Model file for the job. Use its own axes, mm. Give positions to 0.01 mm unless a question says otherwise; leave off trailing zeros. Loops run counter-clockwise (first coordinate to the right, second up) from the corner with the lowest first, then second, coordinate; pieces in that order, holes last. Notation, with made-up numbers: (-23, 56) - (3, 56) arc R26 ccw to (3, 91) - close; hole circle Ø10 at (20.5, -32). An arc over 180 degrees is marked (long way). Answer as CSV lines item,"result". Start each with the question number.
Item 1: Pull direction Y, two halves, no side cores. Call faces 1 (the cylindrical face through (0, -1, 1)), 2 (the flat face through (0, -2, 121)), 3 (the cylindrical face through (0.867, -3.905, 61.34)), 4 (the cylindrical face through (0, -1, 120)): pulls with the +Y half, pulls with the -Y half, needs draft (parallel to the pull), parting line crosses it, or undercut.
Item 2: Pin check, flat tips, straight feed: pin 1 (2 mm diameter, centred on y = 3, z = 22.5, fed in from +X); pin 2 (1 mm diameter, centred on x = -2.5, z = 88.5, fed in from -Y); pin 3 (1 mm diameter, centred on y = -3, z = 99, fed in from -X). Stop position of each tip, or through.
Item 3: Saw through at A-A on z = 64.5. Give the cut face in (x, y), plus the area to 3 significant figures.
Item 4: Drill centre lines: L1, parallel to Y at x = 0, z = 1.15; L2, parallel to Y at x = -0.25, z = 104.5. Where is each one in solid material? Low to high. Write a range as from..to.
from build123d import *

# Parameters (mm, degrees)
CHAMFER1_SIZE         = 0.5
CHAMFER2_SIZE         = 0.3
CHAMFER2_SIZE2        = 0.173205081
CHAMFER2_PART_2_SIZE  = 0.3
CHAMFER2_PART_2_SIZE2 = 0.173205081
CHAMFER2_PART_3_SIZE  = 0.3
CHAMFER2_PART_3_SIZE2 = 0.173205081
CHAMFER2_PART_4_SIZE  = 0.3
CHAMFER2_PART_4_SIZE2 = 0.173205081


with BuildPart() as part:
    # Sketch1 → Revolve1 (revolve)
    with BuildSketch(Plane(origin=(0, 0, 0), x_dir=(1, 0, 0), z_dir=(0, 1, 0))):
        Polygon((-1, 0), (-4, 0), (-4, -121), (-1, -121), (-1, -119), (0, -119), (0, -2), (-1, -2), align=None)
    revolve(axis=Axis((0, 0, 119), (0, 0, -1)))

    # Chamfer1
    chamfer1_edges = [part.edges().sort_by_distance(p)[0] for p in [
        (4, 0, 121),
        (4, 0, 0),
    ]]
    chamfer(chamfer1_edges, length=CHAMFER1_SIZE)

    # Chamfer2
    chamfer2_edges = [part.edges().sort_by_distance(p)[0] for p in [
        (1, 0, 2),
    ]]
    chamfer2_side = [part.faces().sort_by_distance(p)[0] for p in [
        (0, 0, 2),
    ]]
    chamfer(chamfer2_edges, length=CHAMFER2_SIZE, length2=CHAMFER2_SIZE2, reference=chamfer2_side[0])

    # Chamfer2 part 2
    chamfer2_part_2_edges = [part.edges().sort_by_distance(p)[0] for p in [
        (1, 0, 119),
    ]]
    chamfer2_part_2_side = [part.faces().sort_by_distance(p)[0] for p in [
        (1, 0, 120),
    ]]
    chamfer(chamfer2_part_2_edges, length=CHAMFER2_PART_2_SIZE, length2=CHAMFER2_PART_2_SIZE2, reference=chamfer2_part_2_side[0])

    # Chamfer2 part 3
    chamfer2_part_3_edges = [part.edges().sort_by_distance(p)[0] for p in [
        (1, 0, 121),
    ]]
    chamfer2_part_3_side = [part.faces().sort_by_distance(p)[0] for p in [
        (3.401005051, 0, 121),
    ]]
    chamfer(chamfer2_part_3_edges, length=CHAMFER2_PART_3_SIZE, length2=CHAMFER2_PART_3_SIZE2, reference=chamfer2_part_3_side[0])

    # Chamfer2 part 4
    chamfer2_part_4_edges = [part.edges().sort_by_distance(p)[0] for p in [
        (1, 0, 0),
    ]]
    chamfer2_part_4_side = [part.faces().sort_by_distance(p)[0] for p in [
        (1, 0, 1),
    ]]
    chamfer(chamfer2_part_4_edges, length=CHAMFER2_PART_4_SIZE, length2=CHAMFER2_PART_4_SIZE2, reference=chamfer2_part_4_side[0])


solid = part.part
Responses:
1,face 1,"undercut"
1,face 2,"needs draft"
1,face 3,"parting line crosses it"
1,face 4,"undercut"
2,pin 1,"x = 3.46"
2,pin 2,"y = -3.46"
2,pin 3,"x = -3.12"
3,outline,"circle Ø8 at (0, 0)"
3,area,"50.3 mm2"
4,L1,"-4..-1, 1..4"
4,L2,"-3.99..3.99"
